from build123d import *

# Parameters (mm, degrees)
SALIENTE_EXTRUIR1_START       = 0.2
SALIENTE_EXTRUIR1_OUTLINE_R   = 1.802094284
SALIENTE_EXTRUIR1_OUTLINE_R_2 = 1.64762906
SALIENTE_EXTRUIR1_DEPTH       = 3.8
CROQUIS2_R                    = 3.36248758
CROQUIS2_R_2                  = 1.8
SALIENTE_EXTRUIR2_DEPTH       = 6
SIMETR_A5_COPY_1_SKETCH_R     = 3.36248758
SIMETR_A5_COPY_1_SKETCH_R_2   = 1.8
SIMETR_A5_COPY_1_DEPTH        = 6
SIMETR_A5_COPY_2_SKETCH_R     = 3.36248758
SIMETR_A5_COPY_2_SKETCH_R_2   = 1.8
SIMETR_A5_COPY_2_DEPTH        = 6


# Read off the part's stored shape, not the designer's step: Saliente-Extruir1
with BuildPart() as part:
    # Saliente-Extruir1 outline → Saliente-Extruir1 (new body)
    with BuildSketch(Plane.XY.offset(SALIENTE_EXTRUIR1_START)):
        with BuildLine():
            Line((57.990889124, -9.110899758), (86.465185089, 27.016852307))
            ThreePointArc((86.465185089, 27.016852307), (85.905736152, 31.739104142), (81.183484317, 31.179655205))
            Line((81.183484317, 31.179655205), (52.709188351, -4.94809686))
            ThreePointArc((52.709188351, -4.94809686), (53.268637289, -9.670348695), (57.990889124, -9.110899758))
        make_face()
        with Locations((55.350038738, -7.029498309)):
            Circle(SALIENTE_EXTRUIR1_OUTLINE_R, mode=Mode.SUBTRACT)
        with Locations((83.824334703, 29.098253756)):
            Circle(SALIENTE_EXTRUIR1_OUTLINE_R_2, mode=Mode.SUBTRACT)
    saliente_extruir1 = extrude(amount=SALIENTE_EXTRUIR1_DEPTH)

    # Croquis2 → Saliente-Extruir2 (add)
    with BuildSketch(Plane.XY.offset(4)):
        with Locations(Location((55.350038738, -7.029498309, 0), (0, 0, 141.756384729))):
            Circle(CROQUIS2_R)
        with Locations((55.350038738, -7.029498309)):
            Circle(CROQUIS2_R_2, mode=Mode.SUBTRACT)
    saliente_extruir2 = extrude(amount=SALIENTE_EXTRUIR2_DEPTH)

    # Simetría4: Saliente-Extruir2 across plane
    add(saliente_extruir2.mirror(Plane.XY.offset(10)))

    # Simetría5: Saliente-Extruir1 across plane
    add(saliente_extruir1.mirror(Plane.XY.offset(10)))

    # Simetría5 copy 1 sketch → Simetría5 copy 1 (add)
    with BuildSketch(Plane.XY.offset(4)):
        with Locations(Location((55.350038738, -7.029498309, 0), (0, 0, 141.756384729))):
            Circle(SIMETR_A5_COPY_1_SKETCH_R)
        with Locations((55.350038738, -7.029498309)):
            Circle(SIMETR_A5_COPY_1_SKETCH_R_2, mode=Mode.SUBTRACT)
    extrude(amount=SIMETR_A5_COPY_1_DEPTH)

    # Simetría5 copy 2 sketch → Simetría5 copy 2 (add)
    with BuildSketch(Plane(origin=(0, 0, 16), x_dir=(1, 0, 0), z_dir=(0, 0, -1))):
        with Locations((55.350038738, 7.029498309)):
            Circle(SIMETR_A5_COPY_2_SKETCH_R)
        with Locations((55.350038738, 7.029498309)):
            Circle(SIMETR_A5_COPY_2_SKETCH_R_2, mode=Mode.SUBTRACT)
    extrude(amount=SIMETR_A5_COPY_2_DEPTH)


solid = part.part
Model file for the job. Use its own axes, mm. Round coordinates to 2 decimals unless told otherwise and drop trailing zeros. Loops run counter-clockwise (first coordinate to the right, second up) from the corner with the lowest first, then second, coordinate; pieces in that order, holes last.
1. Band-saw the part on C-C, the plane x = 72.5. List the corners of the cut face in (y, z).
Check values:
outline: (9.3, 0.2) - (20.16, 0.2) - (20.16, 4) - (9.3, 4) - close; (9.3, 16) - (20.16, 16) - (20.16, 19.8) - (9.3, 19.8) - close
2. Drop flat-ended pins along their axis: P1, Ø3, axis at x = 55.5, y = -6, coming from the +Z side; P2, Ø8, axis at y = -4, z = 11.5, coming from the +X side; P3, Ø5, axis at y = 3.5, z = 3.5, coming from the +X side; P4, Ø3, axis at x = 67, z = 15.5, coming from the +Y side. Give the stop position or say it passes through.
Check values:
P1: stops at z = 19.8
P2: stops at x = 58.71
P3: stops at x = 69.9
P4: stops at y = 14.98
3. Band-saw the part on B-B, the plane y = 13. List the corners of the cut face in (x, z).
Check values:
outline: (66.86, 0.2) - (75.42, 0.2) - (75.42, 4) - (66.86, 4) - close; (66.86, 16) - (75.42, 16) - (75.42, 19.8) - (66.86, 19.8) - close
4. Band-saw the part on D-D, the plane z = 3.5. List the corners of the cut face in (x, y).
Check values:
outline: (52.71, -4.95) arc R3.36 ccw to (57.99, -9.11) - (86.47, 27.02) arc R3.36 ccw to (81.18, 31.18) - close; hole circle Ø3.6 at (55.35, -7.03); hole circle Ø3.3 at (83.82, 29.1)
5. Band-saw the part on A-A, the plane x = 83.5. List the corners of the cut face in (y, z).
Check values:
outline: (23.25, 0.2) - (27.48, 0.2) - (27.48, 4) - (23.25, 4) - close; (23.25, 16) - (27.48, 16) - (27.48, 19.8) - (23.25, 19.8) - close; (30.71, 0.2) - (32.45, 0.2) - (32.45, 4) - (30.71, 4) - close; (30.71, 16) - (32.45, 16) - (32.45, 19.8) - (30.71, 19.8) - close
6. Wall check: probe 1 along Z at (x, y) = (69.5, 8); probe 2 along Y at (x, z) = (57, 6); probe 3 along X at (y, z) = (-5.5, 7.75). Give the ranges that are in metal, low to high.
Check values:
probe 1: z = 0.2 to 4, 16 to 19.8
probe 2: y = -9.96 to -7.75, -6.31 to -4.1
probe 3: x = 52.36 to 54.4, 56.3 to 58.34
7. Mould opens along Y. For faces 1 (the flat face through (70, 13, 4)), 2 (the flat face through (72.03, 8.7, 2.07)), 3 (the cylindrical face through (57.013, -7.719, 10.084)) say: +Y half, -Y half, draft (parallel to the pull), parting line (faces both ways), or undercut.
Check values:
face 1: draft
face 2: -Y half
face 3: undercut
